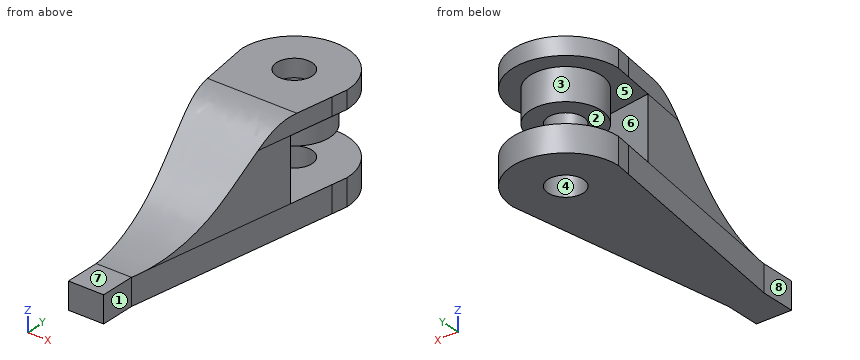
```python
from build123d import *

# Parameters (mm, degrees)
ESQUISSE1_R                  = 5
ESQUISSE1_W                  = 10
ESQUISSE1_H                  = 10
BOSS_EXTRU_1_DEPTH           = 7.5
ESQUISSE2_R                  = 5
BOSS_EXTRU_2_DEPTH           = 5
BOSS_EXTRU_3_DEPTH           = 17.5
ENL_V_MAT_EXTRU_1_DEPTH      = 83.158383626
ENL_V_MAT_EXTRU_1_DEPTH_BACK = 83.158383626
BOSS_EXTRU_4_START           = 9
ESQUISSE5_R                  = 10
ESQUISSE5_R_2                = 5
BOSS_EXTRU_4_DEPTH           = 9


with BuildPart() as part:
    # Esquisse1 → Boss.-Extru.1 (new body)
    # profile 1 of 3: a face of its own
    with BuildSketch(Plane.XY):
        with BuildLine():
            ThreePointArc((14.306358382, -4.50867052), (0, -15), (-14.306358382, -4.50867052))
            Line((-14.306358382, -4.50867052), (-5, -65))
            Line((-5, -65), (5, -65))
            Line((5, -65), (14.306358382, -4.50867052))
        make_face()
    # profile 2 of 3: a face of its own
    with BuildSketch(Plane.XY):
        with BuildLine():
            ThreePointArc((15, 0), (0, 15), (-15, 0))
            Line((-15, 0), (-14.306358382, -4.50867052))
            ThreePointArc((-14.306358382, -4.50867052), (0, -15), (14.306358382, -4.50867052))
            Line((14.306358382, -4.50867052), (15, 0))
        make_face()
        Circle(ESQUISSE1_R, mode=Mode.SUBTRACT)
    # profile 3 of 3: a face of its own
    with BuildSketch(Plane.XY):
        with Locations((0, -70)):
            Rectangle(ESQUISSE1_W, ESQUISSE1_H)
    extrude(amount=BOSS_EXTRU_1_DEPTH)



with BuildPart() as body_2:
    # Esquisse2 → Boss.-Extru.2 (new body)
    # profile 1 of 2: a face of its own
    with BuildSketch(Plane.XY.offset(25)):
        with BuildLine():
            ThreePointArc((14.306358382, -4.50867052), (0, -15), (-14.306358382, -4.50867052))
            Line((-14.306358382, -4.50867052), (-5, -65))
            Line((-5, -65), (5, -65))
            Line((5, -65), (14.306358382, -4.50867052))
        make_face()
    # profile 2 of 2: a face of its own
    with BuildSketch(Plane.XY.offset(25)):
        with BuildLine():
            ThreePointArc((15, 0), (0, 15), (-15, 0))
            Line((-15, 0), (-14.306358382, -4.50867052))
            ThreePointArc((-14.306358382, -4.50867052), (0, -15), (14.306358382, -4.50867052))
            Line((14.306358382, -4.50867052), (15, 0))
        make_face()
        Circle(ESQUISSE2_R, mode=Mode.SUBTRACT)
    extrude(amount=BOSS_EXTRU_2_DEPTH)


with BuildPart() as part_1:
    add(part.part)

    add(body_2.part)  # Boss.-Extru.3 merges body 2
    # Esquisse3 → Boss.-Extru.3 (add)
    with BuildSketch(Plane(origin=(0, 0, 25), x_dir=(-1, 0, 0), z_dir=(0, 0, -1))):
        Polygon((12.972191557, -13.180754881), (-12.372321427, -17.079910725), (-5, -65), (5, -65), align=None)
    extrude(amount=BOSS_EXTRU_3_DEPTH)

    # Esquisse4 → Enlèv. mat.-Extru.1 (cut, two sides: drawn at the far end of the back side and taken through both)
    with BuildSketch(Plane(origin=(0, 0, 0), x_dir=(0, 0, -1), z_dir=(1, 0, 0)).offset(-ENL_V_MAT_EXTRU_1_DEPTH_BACK)):
        with BuildLine():
            Line((-30, -15.176476659), (-30, -65))
            Line((-30, -65), (-7.5, -65))
            add(Edge.make_bspline(
                [(-7.5, -65), (-7.5, -64.789009401), (-5.808728882, -48.116944639), (-22.947732818, -29.702706462), (-30, -20.554677266), (-30, -15.176476659)],
                knots=[0, 0, 0, 0, 0.665017027, 0.876258151, 1, 1, 1, 1], degree=3))
        make_face()
    extrude(amount=ENL_V_MAT_EXTRU_1_DEPTH + ENL_V_MAT_EXTRU_1_DEPTH_BACK, mode=Mode.SUBTRACT)

    # Esquisse5 → Boss.-Extru.4 (add)
    with BuildSketch(Plane(origin=(0, 0, 25), x_dir=(-1, 0, 0), z_dir=(0, 0, -1)).offset(BOSS_EXTRU_4_START)):
        with Locations(Location((0, 0, 0), (0, 0, 180))):
            Circle(ESQUISSE5_R)
        with Locations(Location((0, 0, 0), (0, 0, 180))):
            Circle(ESQUISSE5_R_2, mode=Mode.SUBTRACT)
    extrude(amount=-BOSS_EXTRU_4_DEPTH)


solid = part_1.part
```
Source: CAD feature listing. Evaluate the final solid. Frame: model axes, mm. Face numbers are marked on the shaded views. A direction names the side the tool comes from. Give positions to 0.01 mm unless a question says otherwise; leave off trailing zeros. Write each loop counter-clockwise with the first axis right and the second up, starting at its lowest first coordinate (ties: lowest second). Pieces come first, ordered by that corner, then holes.
1. Section query A-A (y = -1). Return the cut outline in (x, z).
2. Pull-direction query (Z, two-part tool) for the marked faces 5, 6, 7 and 8; classes: +Z half, -Z half, draft (parallel to the pull), parting line (faces both ways), or undercut.
3. Material intervals for line 1 along Z through (x, y) = (0.5, -9); line 2 along Y through (x, z) = (0, 23); line 3 along Y through (x, z) = (0, 21.75), sorted ascending.
4. Section query B-B (z = 6). Return the cut outline in (x, y).
5. Access query for the marked faces 1, 2, 3 and 4. Directions: +Z, -Z, +X, -X, +Y, -Y. A direction counts if a zero-diameter tool reaches every point of the face in a straight line with its end or side. Return the directions, or none.
6. Section query C-C (x = 0). Count the separate pieces of the cut face and the enclosed holes in it, then the cut area to 3 significant figures.
7. First-contact query: pin 1 (10 mm diameter, centred on y = -5, z = 13, fed in from +X); pin 2 (8 mm diameter, centred on y = -69.5, z = 2, fed in from +X); pin 3 (12 mm diameter, centred on x = -11.5, z = 10, fed in from +Y); pin 4 (10 mm diameter, centred on x = 11.5, y = -10.5, fed in from -Z). Flat tips, straight axial feed; report the tip coordinate or a pass-through.
8. Section query D-D (y = -11). Return the cut outline in (x, z).
Output values:
1. outline: (-14.85, 0) - (-4.9, 0) - (-4.9, 7.5) - (-14.85, 7.5) - close; (-14.85, 25) - (-9.95, 25) - (-9.95, 16) - (-4.9, 16) - (-4.9, 30) - (-14.85, 30) - close; (4.9, 0) - (14.85, 0) - (14.85, 7.5) - (4.9, 7.5) - close; (4.9, 16) - (9.95, 16) - (9.95, 25) - (14.85, 25) - (14.85, 30) - (4.9, 30) - close
2. face 5: undercut
2. face 6: undercut
2. face 7: +Z half
2. face 8: draft
3. line 1: z = 0 to 7.5, 16 to 30
3. line 2: y = -29.28 to -15.18, -10 to -5, 5 to 10
3. line 3: y = -30.77 to -15.18, -10 to -5, 5 to 10
4. outline: (-15, 0) - (-5, -65) - (-5, -75) - (5, -75) - (5, -65) - (15, 0) arc R15 ccw to start; hole circle Ø10 at (0, 0)
5. face 1: +Z, -Z, +X, -Y
5. face 2: +X, -X, +Y
5. face 3: none
5. face 4: +Z, -Z
6. separate pieces: 3
6. enclosed holes: 0
6. area: 1,240 mm2
7. pin 1: stops at x = 9.95
7. pin 2: stops at x = 5
7. pin 3: stops at y = 13.73
7. pin 4: stops at z = 0
8. outline: (-13.31, 0) - (13.31, 0) - (13.31, 7.5) - (-13.31, 7.5) - close; (-13.31, 25) - (13.31, 25) - (13.31, 30) - (-13.31, 30) - close
